Geometry: see drawing. Coordinates: mm, zero at the bounding-box minimum. A direction names the side the tool comes from. Give positions to 0.01 mm unless a question says otherwise; leave off trailing zeros. Write each loop counter-clockwise with the first axis right and the second up, starting at its lowest first coordinate (ties: lowest second). Pieces come first, ordered by that corner, then holes. Notation, with made-up numbers: (86.25, -32.5) -> (126.25, -32.5) arc R11 ccw to (126.25, -12.5) -> close; hole circle Ø5 at (68.25, 7). An arc over 180 degrees is marked (long way). Write item = value, one per line.
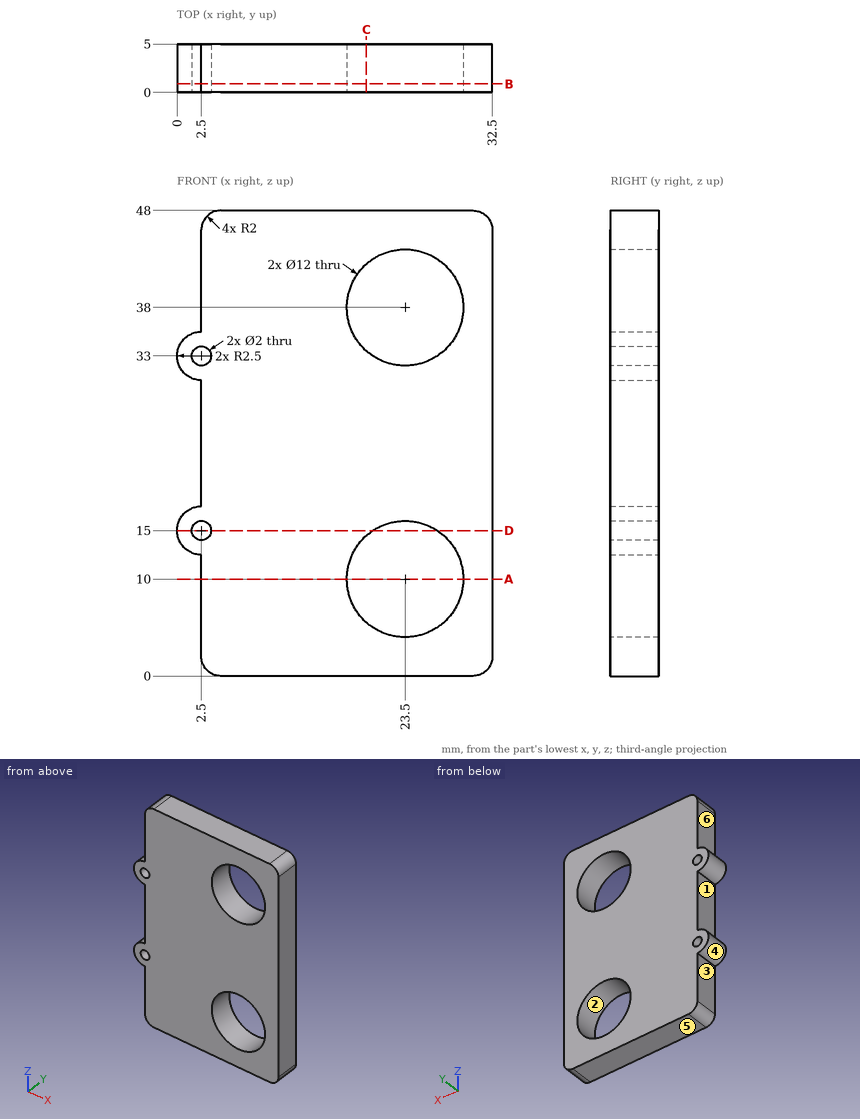
(1) Section query D-D (z = 15). Return loops of the section in (x, y).
Values follow:
outline = (0, 0) -> (1.5, 0) -> (1.5, 5) -> (0, 5) -> close; (3.5, 0) -> (20.18, 0) -> (20.18, 5) -> (3.5, 5) -> close; (26.82, 0) -> (32.5, 0) -> (32.5, 5) -> (26.82, 5) -> close
(2) Section query C-C (x = 19.5). Return loops of the section in (y, z), plus the area to 3 significant figures.
Values follow:
outline = (0, 0) -> (5, 0) -> (5, 5.53) -> (0, 5.53) -> close; (0, 14.47) -> (5, 14.47) -> (5, 33.53) -> (0, 33.53) -> close; (0, 42.47) -> (5, 42.47) -> (5, 48) -> (0, 48) -> close
area = 151 mm2
(3) First-contact query: pin 1 (2.5 mm diameter, centred on y = 1.5, z = 42, fed in from -X); pin 2 (1.6 mm diameter, centred on x = 2.5, z = 33, fed in from -Y). Flat tips, straight axial feed; report the tip coordinate or a pass-through.
Values follow:
pin_1 = 2.5
pin_2 = through
(4) Section query B-B (y = 0.9). Return loops of the section in (x, z), plus the area to 3 significant figures.
Values follow:
outline = (2.5, 2) arc R2 ccw to (4.5, 0) -> (30.5, 0) arc R2 ccw to (32.5, 2) -> (32.5, 46) arc R2 ccw to (30.5, 48) -> (4.5, 48) arc R2 ccw to (2.5, 46) -> (2.5, 35.5) arc R2.5 ccw to (2.5, 30.5) -> (2.5, 17.5) arc R2.5 ccw to (2.5, 12.5) -> close; hole circle Ø2 at (2.5, 15); hole circle Ø2 at (2.5, 33); hole circle Ø12 at (23.5, 10); hole circle Ø12 at (23.5, 38)
area = 1,220 mm2
(5) Access query for the marked faces 1, 2 and 3. Directions: +Z, -Z, +X, -X, +Y, -Y. A direction counts if a zero-diameter tool reaches every point of the face in a straight line with its end or side. Return the directions, or none.
Values follow:
face_1 = -X, +Y, -Y
face_2 = +Y, -Y
face_3 = -Z, -X, +Y, -Y
(6) Material intervals for line 1 (X direction, y = 2.85, z = 15); line 2 (X direction, y = 2.6, z = 10); line 3 (Z direction, x = 2, y = 2.6), sorted ascending.
Values follow:
line_1 = 0 to 1.5, 3.5 to 20.18, 26.82 to 32.5
line_2 = 2.5 to 17.5, 29.5 to 32.5
line_3 = 12.55 to 14.13, 15.87 to 17.45, 30.55 to 32.13, 33.87 to 35.45
(7) Pull-direction query (Z, two-part tool) for the marked faces 4, 5 and 6; classes: pulls with the +Z half, pulls with the -Z half, needs draft (parallel to the pull), parting line crosses it, or undercut.
Values follow:
face_4 = undercut
face_5 = pulls with the -Z half
face_6 = needs draft
(8) Section query A-A (z = 10). Return loops of the section in (x, y), plus the area to 3 significant figures.
Values follow:
outline = (2.5, 0) -> (17.5, 0) -> (17.5, 5) -> (2.5, 5) -> close; (29.5, 0) -> (32.5, 0) -> (32.5, 5) -> (29.5, 5) -> close
area = 90.0 mm2
